Geometry: final body of the model. Coordinates: model frame, mm. Give positions to 0.01 mm unless a question says otherwise; leave off trailing zeros. Order: outer loops, then holes, each group sorted by start corner. A loop starts at its lowest first (then second) coordinate and runs counter-clockwise, first axis right, second up. Notation, with made-up numbers: (-33.5, 58.5) - (-27.5, 58.5) arc R35 cw to (-27.5, 97.5) - close; hole circle Ø6 at (85.5, 69.25). An arc over 180 degrees is marked (long way). One line per item, written item: value.
```python
from build123d import *

# Parameters (mm, degrees)
F0_W     = 3
F0_H     = 5
F0_W_2   = 1.5
F0_H_2   = 3
F1_DEPTH = 3


with BuildPart() as f1:
    # F0 (on Front) → F1 (new body)
    with BuildSketch(Plane.XZ):
        Polygon((1.5, 5), (1.5, 0), (4.5, 0), (4.5, -2), (11.5, -2), (11.5, 0), (14.5, 0), (14.5, 5), (14.5, 10), (11.5, 10), (1.5, 10), align=None)
        with Locations((16, 2.5)):
            Rectangle(F0_W, F0_H)
        Polygon((20.5, 10), (17.5, 10), (17.5, 5), (17.5, 0), (30.5, 0), (30.5, 5), (30.5, 10), align=None)
        with Locations((32, 2.5)):
            Rectangle(F0_W, F0_H)
        Polygon((33.5, 5), (33.5, 0), (36.5, 0), (36.5, -2), (43.5, -2), (43.5, 0), (48, 0), (52.5, 0), (52.5, -2), (59.5, -2), (59.5, 0), (62.5, 0), (62.5, 5), (62.5, 10), (33.5, 10), align=None)
        with Locations((64, 2.5)):
            Rectangle(F0_W, F0_H)
        Polygon((78.5, 10), (65.5, 10), (65.5, 5), (65.5, 0), (78.5, 0), (78.5, 5), align=None)
        with Locations((80, 2.5)):
            Rectangle(F0_W, F0_H)
        Polygon((110.5, 10), (81.5, 10), (81.5, 5), (81.5, 0), (84.5, 0), (84.5, -2), (91.5, -2), (91.5, 0), (96, 0), (100.5, 0), (100.5, -2), (107.5, -2), (107.5, 0), (110.5, 0), (110.5, 5), align=None)
        with Locations((112, 2.5)):
            Rectangle(F0_W, F0_H)
        Polygon((126.5, 10), (113.5, 10), (113.5, 5), (113.5, 0), (126.5, 0), (126.5, 5), align=None)
        with Locations((128, 2.5)):
            Rectangle(F0_W, F0_H)
        Polygon((158.5, 10), (129.5, 10), (129.5, 5), (129.5, 0), (132.5, 0), (132.5, -2), (139.5, -2), (139.5, 0), (144, 0), (148.5, 0), (148.5, -2), (155.5, -2), (155.5, 0), (158.5, 0), (158.5, 5), align=None)
        with Locations((160, 2.5)):
            Rectangle(F0_W, F0_H)
        Polygon((171.5, 10), (161.5, 10), (161.5, 5), (161.5, 0), (174.5, 0), (174.5, 5), (174.5, 10), align=None)
        with Locations((176, 2.5)):
            Rectangle(F0_W, F0_H)
        Polygon((180.5, 10), (177.5, 10), (177.5, 5), (177.5, 0), (180.5, 0), (180.5, -2), (187.5, -2), (187.5, 0), (190.5, 0), (190.5, 5), (190.5, 10), align=None)
        with Locations((0.75, 2.5)):
            Rectangle(F0_W_2, F0_H)
        with Locations((191.25, 2.5)):
            Rectangle(F0_W_2, F0_H)
        with Locations((192.75, 2.5)):
            Rectangle(F0_W_2, F0_H)
        with Locations((-0.75, 2.5)):
            Rectangle(F0_W_2, F0_H)
        with Locations((173, 11.5)):
            Rectangle(F0_W, F0_H_2)
        with Locations((179, 11.5)):
            Rectangle(F0_W, F0_H_2)
        with Locations((19, 11.5)):
            Rectangle(F0_W, F0_H_2)
        with Locations((13, 11.5)):
            Rectangle(F0_W, F0_H_2)
    extrude(amount=F1_DEPTH)


solid = f1.part
```
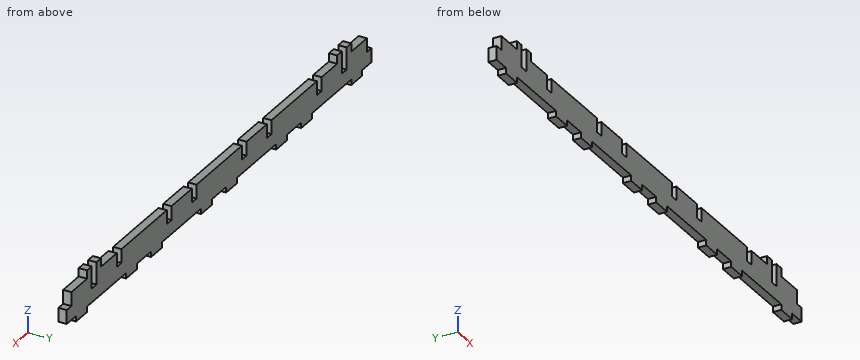
1) First-contact query: pin 1 (1 mm diameter, centred on y = -1, z = -1.5, fed in from -X); pin 2 (0.6 mm diameter, centred on y = -1.5, z = -1, fed in from +X); pin 3 (2 mm diameter, centred on x = 83.5, z = 10.5, fed in from -Y); pin 4 (1.5 mm diameter, centred on x = 112.5, y = -1.5, fed in from +Z). Flat tips, straight axial feed; report the tip coordinate or a pass-through.
Answers below:
pin 1: x = 4.5
pin 2: x = 187.5
pin 3: y = -3
pin 4: z = 5
2) Section B-B, the plane x = 49.5. Return loops of the section in (y, z).
Answers below:
outline: (-3, 0) - (0, 0) - (0, 10) - (-3, 10) - close
3) Section A-A, the plane x = 136. Return loops of the section in (y, z).
Answers below:
outline: (-3, -2) - (0, -2) - (0, 10) - (-3, 10) - close
4) Material intervals for line 1 along X through (y, z) = (-1.15, 10.5); line 2 along Z through (x, y) = (130, -1.4); line 3 along Z through (x, y) = (32.5, -0.3), sorted ascending.
Answers below:
line 1: 11.5 to 14.5, 17.5 to 20.5, 171.5 to 174.5, 177.5 to 180.5
line 2: 0 to 10
line 3: 0 to 5
